The listing builds one solid part. Answer for the finished solid, in the listing's coordinates (mm). A direction names the side the tool comes from. Coordinates: 2 decimals unless noted, no trailing zeros. Order: outer loops, then holes, each group sorted by start corner. A loop starts at its lowest first (then second) coordinate and runs counter-clockwise, first axis right, second up. Notation, with made-up numbers: (-8, -1.75) - (37, -1.75) arc R21 ccw to (37, 19.25) - close; hole circle Ø7 at (5, -32). An arc over 180 degrees is marked (long way). One line per item, written item: value. Start each with the question number.
```python
from build123d import *

# Parameters (mm, degrees)
SKETCH_1_R               = 16
EXTRUDE_1_DEPTH          = 2.4
SKETCH_2_R               = 7
EXTRUDE_2_DEPTH          = 6.4
CUT_EXTRUDE_1_REACH      = 26.278
SKETCH_3_R               = 3
CUT_EXTRUDE_2_REACH      = 25.515
SKETCH_4_R               = 2.1
CUT_EXTRUDE_3_REACH      = 26.278
CUT_EXTRUDE_3_END_RADIUS = 7
SKETCH_5_R               = 1.5


with BuildPart() as part:
    # 草圖1 → 填料-伸長1 (new body)
    with BuildSketch(Plane(origin=(0, 0, 0), x_dir=(1, 0, 0), z_dir=(0, 1, 0))):
        with Locations(Location((0, 0, 0), (0, 0, 270))):
            Circle(SKETCH_1_R)
    extrude(amount=EXTRUDE_1_DEPTH)

    # 草圖2 → 填料-伸長2 (add)
    with BuildSketch(Plane(origin=(0, 2.4, 0), x_dir=(1, 0, 0), z_dir=(0, 1, 0))):
        with Locations(Location((0, 0, 0), (0, 0, 270))):
            Circle(SKETCH_2_R)
    extrude(amount=EXTRUDE_2_DEPTH)

    # 草圖3 → 除料-伸長1 (cut, up to next)
    with BuildSketch(Plane(origin=(0, 8.8, 0), x_dir=(1, 0, 0), z_dir=(0, 1, 0)), mode=Mode.PRIVATE) as cut_extrude_1_sk1:
        with Locations(Location((0, 0, 0), (0, 0, 270))):
            Circle(SKETCH_3_R)
    cut_extrude_1_tool1 = extrude(cut_extrude_1_sk1.sketch, amount=-CUT_EXTRUDE_1_REACH, mode=Mode.PRIVATE) & part.part
    add(cut_extrude_1_tool1.solids().sort_by_distance((0, 8.8, 0))[0], mode=Mode.SUBTRACT)

    # 草圖4 → 除料-伸長2 (cut, up to next)
    with BuildSketch(Plane(origin=(0, 2.4, 0), x_dir=(1, 0, 0), z_dir=(0, 1, 0)), mode=Mode.PRIVATE) as cut_extrude_2_sk1:
        with Locations(Location((0, 11.29, 0), (0, 0, 270))):
            Circle(SKETCH_4_R)
    cut_extrude_2_tool1 = extrude(cut_extrude_2_sk1.sketch, amount=-CUT_EXTRUDE_2_REACH, mode=Mode.PRIVATE) & part.part
    # 草圖4 → 除料-伸長2 (cut, up to next)
    with BuildSketch(Plane(origin=(0, 2.4, 0), x_dir=(1, 0, 0), z_dir=(0, 1, 0)), mode=Mode.PRIVATE) as cut_extrude_2_sk2:
        with Locations(Location((11.29, 0, 0), (0, 0, 270))):
            Circle(SKETCH_4_R)
    cut_extrude_2_tool2 = extrude(cut_extrude_2_sk2.sketch, amount=-CUT_EXTRUDE_2_REACH, mode=Mode.PRIVATE) & part.part
    # 草圖4 → 除料-伸長2 (cut, up to next)
    with BuildSketch(Plane(origin=(0, 2.4, 0), x_dir=(1, 0, 0), z_dir=(0, 1, 0)), mode=Mode.PRIVATE) as cut_extrude_2_sk3:
        with Locations(Location((0, -11.29, 0), (0, 0, 270))):
            Circle(SKETCH_4_R)
    cut_extrude_2_tool3 = extrude(cut_extrude_2_sk3.sketch, amount=-CUT_EXTRUDE_2_REACH, mode=Mode.PRIVATE) & part.part
    # 草圖4 → 除料-伸長2 (cut, up to next)
    with BuildSketch(Plane(origin=(0, 2.4, 0), x_dir=(1, 0, 0), z_dir=(0, 1, 0)), mode=Mode.PRIVATE) as cut_extrude_2_sk4:
        with Locations(Location((-11.29, 0, 0), (0, 0, 270))):
            Circle(SKETCH_4_R)
    cut_extrude_2_tool4 = extrude(cut_extrude_2_sk4.sketch, amount=-CUT_EXTRUDE_2_REACH, mode=Mode.PRIVATE) & part.part
    add(cut_extrude_2_tool1.solids().sort_by_distance((0, 2.4, -11.29))[0], mode=Mode.SUBTRACT)
    add(cut_extrude_2_tool2.solids().sort_by_distance((11.29, 2.4, 0))[0], mode=Mode.SUBTRACT)
    add(cut_extrude_2_tool3.solids().sort_by_distance((0, 2.4, 11.29))[0], mode=Mode.SUBTRACT)
    add(cut_extrude_2_tool4.solids().sort_by_distance((-11.29, 2.4, 0))[0], mode=Mode.SUBTRACT)

    # 除料-伸長3: up to this cylinder (the profile starts inside it)
    cut_extrude_3_end = Plane(origin=(0, 5.6, 0), z_dir=(0, -1, 0)) * Cylinder(CUT_EXTRUDE_3_END_RADIUS, 67.556, mode=Mode.PRIVATE)
    # 草圖5 → 除料-伸長3 (cut, up to the surface)
    with BuildSketch(Plane.XY, mode=Mode.PRIVATE) as cut_extrude_3_sk1:
        with Locations(Location((0, 5.6, 0), (0, 0, 180))):
            Circle(SKETCH_5_R)
    cut_extrude_3_tool1 = extrude(cut_extrude_3_sk1.sketch, amount=CUT_EXTRUDE_3_REACH, mode=Mode.PRIVATE) & cut_extrude_3_end
    add(cut_extrude_3_tool1.solids().sort_by_distance((0, 5.6, 0))[0], mode=Mode.SUBTRACT)


solid = part.part
```
(1) For faces 4 (the face through (9.24, 1.22, -0.46)), 5 (the face through (-3, 2.4, 7)), determine the directions among +Z, -Z, +X, -X, +Y, -Y from which every point of the face is accessible in a straight line to the end or side of a thin tool.
(2) Flat-ended cylindrical pins translate along their axes: pin 1 Ø4 at (y, z) = (1, 1.5) entering from -X; pin 2 Ø3 at (x, y) = (-4.5, 1) entering from -Z; pin 3 Ø2 at (x, z) = (2, -9.5) entering from +Y; pin 4 Ø1 at (y, z) = (2.5, -7.5) entering from -X. Find the tip coordinate at first contact, or state that the pin passes through.
(3) For a pull along Z with two mould halves and no side action, classify faces 1 (the face through (-15.62, 1.18, -3.47)), 2 (the face through (0.631, 1.217, -9.287)), 3 (the face through (1.5, 5.53, 4.77)) as pulls with the +Z half, pulls with the -Z half, needs draft (parallel to the pull), parting line crosses it, or undercut.
(4) The part is cut by section D-D on z = -12. Determine the outline of the cut face in (x, y).
(5) The part is cut by section C-C on x = -10. Determine the outline of the cut face in (y, z), plus the area to 3 significant figures.
(6) The part is cut by section A-A on x = 0. Determine the outline of the cut face in (y, z), plus the area to 3 significant figures.
(7) Consider probe 1 along X at (y, z) = (1.15, 0); probe 2 along X at (y, z) = (4.75, 0); probe 3 along Y at (x, z) = (-8.5, -9.5). Determine where each line is inside the solid, lowest interval first.
(8) The part is cut by section B-B on z = 0. Determine the outline of the cut face in (x, y), plus the area to 3 significant figures.
Completed:
1. face 4: +Y, -Y
1. face 5: +Y
2. pin 1: stops at x = -16
2. pin 2: stops at z = -15.72
2. pin 3: stops at y = 2.4
2. pin 4: stops at x = -14.38
3. face 1: parting line crosses it
3. face 2: undercut
3. face 3: needs draft
4. outline: (-10.58, 0) - (-1.98, 0) - (-1.98, 2.4) - (-10.58, 2.4) - close; (1.98, 0) - (10.58, 0) - (10.58, 2.4) - (1.98, 2.4) - close
5. outline: (0, -12.49) - (2.4, -12.49) - (2.4, -1.66) - (0, -1.66) - close; (0, 1.66) - (2.4, 1.66) - (2.4, 12.49) - (0, 12.49) - close
5. area: 52.0 mm2
6. outline: (0, -16) - (2.4, -16) - (2.4, -13.39) - (0, -13.39) - close; (0, -9.19) - (2.4, -9.19) - (2.4, -7) - (8.8, -7) - (8.8, -3) - (0, -3) - close; (0, 3) - (4.1, 3) - (4.1, 7) - (2.4, 7) - (2.4, 9.19) - (0, 9.19) - close; (0, 13.39) - (2.4, 13.39) - (2.4, 16) - (0, 16) - close; (7.1, 3) - (8.8, 3) - (8.8, 7) - (7.1, 7) - close
6. area: 81.4 mm2
7. probe 1: x = -16 to -13.39, -9.19 to -3, 3 to 9.19, 13.39 to 16
7. probe 2: x = -7 to -3, 3 to 7
7. probe 3: y = 0 to 2.4
8. outline: (-16, 0) - (-13.39, 0) - (-13.39, 2.4) - (-16, 2.4) - close; (-9.19, 0) - (-3, 0) - (-3, 8.8) - (-7, 8.8) - (-7, 2.4) - (-9.19, 2.4) - close; (3, 0) - (9.19, 0) - (9.19, 2.4) - (7, 2.4) - (7, 8.8) - (3, 8.8) - close; (13.39, 0) - (16, 0) - (16, 2.4) - (13.39, 2.4) - close
8. area: 93.4 mm2
